Geometry: final body of the model. Coordinates: model frame, mm. Round coordinates to 2 decimals unless told otherwise and drop trailing zeros. Loops run counter-clockwise (first coordinate to the right, second up) from the corner with the lowest first, then second, coordinate; pieces in that order, holes last. Notation, with made-up numbers: (89.25, 67.25) - (125.25, 67.25) arc R19 cw to (125.25, 101.25) - close; hole circle Ø2 at (59, 4.25). An arc over 180 degrees is marked (long way). Use CSV: the item, a comma, the result in double quotes.
from build123d import *

# Parameters (mm, degrees)
SKIZZE1_W                            = 15
SKIZZE1_H                            = 15
SKIZZE1_R                            = 1.6
AUFSATZ_LINEAR_AUSTRAGEN1_DEPTH      = 6
SCHNITT_LINEAR_AUSTRAGEN1_DEPTH      = 13.186057607
SCHNITT_LINEAR_AUSTRAGEN1_DEPTH_BACK = 13.186057607
SKIZZE2_R                            = 3.1
VERRUNDUNG1_R                        = 3


with BuildPart() as part:
    # Skizze1 → Aufsatz-Linear austragen1 (new body)
    with BuildSketch(Plane.XY):
        Rectangle(SKIZZE1_W, SKIZZE1_H)
        with Locations((5, 5)):
            Circle(SKIZZE1_R, mode=Mode.SUBTRACT)
        with Locations((-5, 5)):
            Circle(SKIZZE1_R, mode=Mode.SUBTRACT)
        with Locations((-5, -5)):
            Circle(SKIZZE1_R, mode=Mode.SUBTRACT)
        with Locations((5, -5)):
            Circle(SKIZZE1_R, mode=Mode.SUBTRACT)
    extrude(amount=-AUFSATZ_LINEAR_AUSTRAGEN1_DEPTH)

    # Skizze2 → Schnitt-Linear austragen1 (cut, two sides: drawn at the far end of the back side and taken through both)
    with BuildSketch(Plane(origin=(0, 0, 0), x_dir=(1, 0, 0), z_dir=(0, 1, 0)).offset(-SCHNITT_LINEAR_AUSTRAGEN1_DEPTH_BACK)):
        Circle(SKIZZE2_R)
    extrude(amount=SCHNITT_LINEAR_AUSTRAGEN1_DEPTH + SCHNITT_LINEAR_AUSTRAGEN1_DEPTH_BACK, mode=Mode.SUBTRACT)

    # Verrundung1
    verrundung1_edges = [part.edges().sort_by_distance(p)[0] for p in [
        (-7.5, 7.5, -3),
        (7.5, 7.5, -3),
        (7.5, -7.5, -3),
        (-7.5, -7.5, -3),
    ]]
    fillet(verrundung1_edges, radius=VERRUNDUNG1_R)


solid = part.part
Item 1: Section B-B on z = -5.15. Return the cut outline in (x, y), plus the area to 3 significant figures.
Final values:
outline,"(-7.5, -4.5) arc R3 ccw to (-4.5, -7.5) - (4.5, -7.5) arc R3 ccw to (7.5, -4.5) - (7.5, 4.5) arc R3 ccw to (4.5, 7.5) - (-4.5, 7.5) arc R3 ccw to (-7.5, 4.5) - close; hole circle Ø3.2 at (-5, -5); hole circle Ø3.2 at (-5, 5); hole circle Ø3.2 at (5, -5); hole circle Ø3.2 at (5, 5)"
area,"185 mm²"
Item 2: Pin query (flat end, axial travel): P1, Ø2.5, axis at x = -5, y = -5, coming from the -Z side; P2, Ø1, axis at y = 5.5, z = -1, coming from the +X side; P3, Ø4, axis at x = 5, y = 5, coming from the -Z side. Return the tip coordinate at first contact, or that it passes through.
Final values:
P1,"passes through"
P2,"stops at x = 7.46"
P3,"stops at z = -6"
Item 3: Section A-A on z = -0.5. Return the cut outline in (x, y), plus the area to 3 significant figures.
Final values:
outline,"(-7.5, -4.5) arc R3 ccw to (-4.5, -7.5) - (-3.06, -7.5) - (-3.06, 7.5) - (-4.5, 7.5) arc R3 ccw to (-7.5, 4.5) - close; (3.06, -7.5) - (4.5, -7.5) arc R3 ccw to (7.5, -4.5) - (7.5, 4.5) arc R3 ccw to (4.5, 7.5) - (3.06, 7.5) - close; hole circle Ø3.2 at (-5, -5); hole circle Ø3.2 at (-5, 5); hole circle Ø3.2 at (5, -5); hole circle Ø3.2 at (5, 5)"
area,"93.3 mm²"
Item 4: Section C-C on x = -5.5. Return the cut outline in (y, z).
Final values:
outline,"(-7.33, -6) - (-6.52, -6) - (-6.52, 0) - (-7.33, 0) - close; (-3.48, -6) - (3.48, -6) - (3.48, 0) - (-3.48, 0) - close; (6.52, -6) - (7.33, -6) - (7.33, 0) - (6.52, 0) - close"
Item 5: Mould query, pull axis X, two halves, no side actions, for faces 1 (the cylindrical face through (6.6, 6.64, -3.04)), 2 (the cylindrical face through (-6.27, 4.03, -2.96)), 3 (the cylindrical face through (-6.6, -4.93, -2.96)), 4 (the flat face through (0, 7.5, -4)). Classes: released by +X, released by -X, zero draft, split by the parting line, or undercut.
Final values:
face 1,"released by +X"
face 2,"undercut"
face 3,"undercut"
face 4,"zero draft"
Item 6: Material intervals for line 1 (Y direction, x = -5, z = -4.05); line 2 (X direction, y = 4.75, z = -1.55); line 3 (X direction, y = -4, z = -4.35), sorted ascending.
Final values:
line 1,"y = -7.46 to -6.6, -3.4 to 3.4, 6.6 to 7.46"
line 2,"x = -7.49 to -6.58, -3.42 to -2.68, 2.68 to 3.42, 6.58 to 7.49"
line 3,"x = -7.5 to -6.25, -3.75 to 3.75, 6.25 to 7.5"
Item 7: Section D-D on y = -0.75. Return the cut outline in (x, z).
Final values:
outline,"(-7.5, -6) - (7.5, -6) - (7.5, 0) - (3.1, 0) arc R3.1 cw to (-3.1, 0) - (-7.5, 0) - close"
